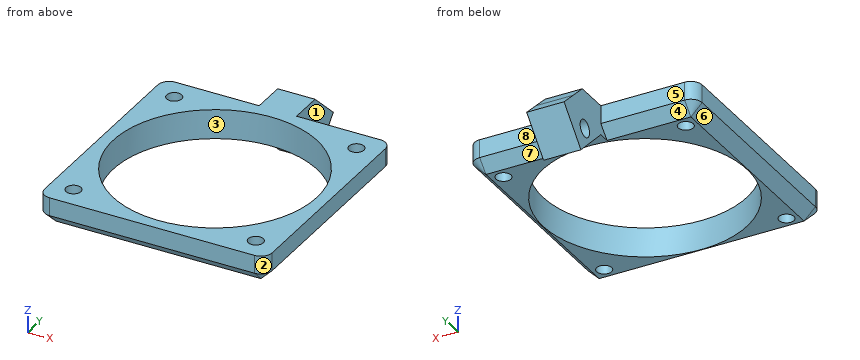
```python
from build123d import *

# Parameters (mm, degrees)
F0_W     = 40.2
F0_H     = 40.2
F0_R     = 1.325
F0_R_2   = 18
F1_DEPTH = 5.2
F2_R     = 2
F6_DEPTH = 3.3
F7_SIZE  = 1.99999


# Not quite as in the source:
# - a fillet or chamfer is up to 0.001 mm smaller than in the source, because OpenCascade refuses the exact size


with BuildPart() as f1:
    # F0 (on Top) → F1 (new body)
    with BuildSketch(Plane.XY):
        Rectangle(F0_W, F0_H)
        with Locations((-16.1, -16.1)):
            Circle(F0_R, mode=Mode.SUBTRACT)
        with Locations((16.1, -16.1)):
            Circle(F0_R, mode=Mode.SUBTRACT)
        with Locations((-16.1, 16.1)):
            Circle(F0_R, mode=Mode.SUBTRACT)
        Circle(F0_R_2, mode=Mode.SUBTRACT)
        with Locations((16.1, 16.1)):
            Circle(F0_R, mode=Mode.SUBTRACT)
    extrude(amount=F1_DEPTH)

    # F2
    f2_edges = [f1.edges().sort_by_distance(p)[0] for p in [
        (-20.1, 20.1, 2.6),
        (20.1, 20.1, 2.6),
        (20.1, -20.1, 2.6),
        (-20.1, -20.1, 2.6),
    ]]
    fillet(f2_edges, radius=F2_R)

    # F5 (on line) → F6 (join, symmetric)
    with BuildSketch(Plane.YZ):
        Polygon((20.1, 5.2), (20.1, 0), (26.4531082501, -5.9914017233), (31.8527851563, -0.1601095172), (28.929274422, 2.5199452414), (26.0057636878, 5.2), align=None)
        with BuildLine():
            ThreePointArc((26.7126609223, -1.5342851533), (23.8396290954, -2.1382583334), (26.2262827859, -0.4285859547))
            ThreePointArc((26.2262827859, -0.4285859547), (26.5856927492, -0.9303119732), (26.7126609223, -1.5342851533))
        make_face(mode=Mode.SUBTRACT)
    extrude(amount=F6_DEPTH, both=True)

    # F7 (size 2 in the source; OpenCascade refuses exactly that, so slightly less here)
    f7_edges = [f1.edges().sort_by_distance(p)[0] for p in [
        (0, -20.1, 0),
    ]]
    chamfer(f7_edges, length=F7_SIZE)


solid = f1.part
```
For this review, take the finished solid that the model builds, in its own axes (mm). Face numbers are marked on the shaded views. A direction names the side the tool comes from. Round coordinates to 2 decimals unless told otherwise and drop trailing zeros. Write each loop counter-clockwise with the first axis right and the second up, starting at its lowest first coordinate (ties: lowest second). Pieces come first, ordered by that corner, then holes. Notation, with made-up numbers: (23.25, -28.5) -> (37.25, -28.5) arc R27 cw to (37.25, 5.5) -> close; hole circle Ø7 at (5.25, 76.5). An arc over 180 degrees is marked (long way). Use one line per item in the form item = value.
Q1. Consider section D-D (x = -8). State the section outline as (y, z) points, then the cut area to 3 significant figures.
Resolved:
outline = (-20.1, 2) -> (-18.1, 0) -> (-16.12, 0) -> (-16.12, 5.2) -> (-20.1, 5.2) -> close; (16.12, 0) -> (18.1, 0) -> (20.1, 2) -> (20.1, 5.2) -> (16.12, 5.2) -> close
area = 37.3 mm²
Q2. The part is to be moulded in two halves that separate along Y. For the marked faces 1, 2 and 3, say which applies: released by +Y, released by -Y, zero draft, split by the parting line, or undercut.
Resolved:
face_1 = zero draft
face_2 = released by -Y
face_3 = undercut
Q3. Machinability: for the marked faces 4, 5, 6, 7 and 8, which of the approach directions +Z, -Z, +X, -X, +Y, -Y give a long, thin tool a straight path to every point of the face, cutting with its end or side? Answer none if there is none.
Resolved:
face_4 = -Z, -X, +Y
face_5 = +Z, -Z, -X, +Y
face_6 = -Z, -X, +Y, -Y
face_7 = -Z, +X, +Y
face_8 = +Z, -Z, +X, +Y
Q4. To check wall thickness, follow probe 1 along Y at (x, z) = (-16.1, 2.05) (3 decimals); probe 2 along Y at (x, z) = (-16.1, 1.1) (3 decimals); probe 3 along Z at (x, y) = (-12, 16). State the ranges of each line that lie inside material, in increasing order. Write a range as from..to.
Resolved:
probe_1 = -20.1..-17.425, -14.775..-8.049, 8.049..14.775, 17.425..20.1
probe_2 = -19.2..-17.425, -14.775..-8.049, 8.049..14.775, 17.425..19.2
probe_3 = 0..5.2
Q5. Consider section C-C (z = -1). State the section outline as (x, y) points.
Resolved:
outline = (-3.3, 21.16) -> (3.3, 21.16) -> (3.3, 23.81) -> (-3.3, 23.81) -> close; (-3.3, 26.61) -> (3.3, 26.61) -> (3.3, 31.08) -> (-3.3, 31.08) -> close
Q6. Consider section A-A (x = 0). State the section outline as (y, z) points.
Resolved:
outline = (-20.1, 2) -> (-18.1, 0) -> (-18, 0) -> (-18, 5.2) -> (-20.1, 5.2) -> close; (18, 0) -> (20.1, 0) -> (26.45, -5.99) -> (31.85, -0.16) -> (26.01, 5.2) -> (18, 5.2) -> close; hole circle Ø3 at (25.21, -1.53)
Q7. Clearance check with flat-ended pins moving along their axes: pin 1 Ø4 at (y, z) = (25.21, -1.53) entering from -X; pin 2 Ø10 at (x, y) = (6.5, -8.5) entering from -Z; pin 3 Ø5 at (y, z) = (-12, -1.5) entering from -X; pin 4 Ø2.5 at (x, z) = (-13, 3) entering from +Y. State where each tip first meets the part, or that it passes through.
Resolved:
pin_1 = -3.3
pin_2 = through
pin_3 = -19.1
pin_4 = 20.1
Q8. Consider section B-B (y = 0). State the section outline as (x, z) points.
Resolved:
outline = (-20.1, 2) -> (-18.1, 0) -> (-18, 0) -> (-18, 5.2) -> (-20.1, 5.2) -> close; (18, 0) -> (18.1, 0) -> (20.1, 2) -> (20.1, 5.2) -> (18, 5.2) -> close
